Part model, mm, in its own coordinate system. Face numbers are marked on the shaded views. A direction names the side the tool comes from. Round coordinates to 2 decimals unless told otherwise and drop trailing zeros. Loops run counter-clockwise (first coordinate to the right, second up) from the corner with the lowest first, then second, coordinate; pieces in that order, holes last.
(1) Cut at B-B on z = -49. List the corners of the cut face in (x, y).
(2) Tool access for the marked faces 1 and 2: list every direction of +Z, -Z, +X, -X, +Y, -Y with a clear straight run to the whole face (end or side of a thin tool).
(3) Probe probe 1 along Z at (x, y) = (11.5, -2.75); probe 2 along Z at (x, y) = (1.5, -7.75); probe 3 along Y at (x, z) = (7.5, -108). List the from-to ranges inside material, lowest first.
(4) Flat gauge pins, fed straight in: pin 1 (4 mm diameter, centred on y = -9, z = -31.5, fed in from +X); pin 2 (2.5 mm diameter, centred on x = 6.5, y = 2.5, fed in from -Z); pin 3 (1 mm diameter, centred on y = -2.5, z = -69.5, fed in from -X); pin 4 (4 mm diameter, centred on x = 9.5, z = -116, fed in from +Y). Where does each tip first touch, or does it go through?
(5) Cut at C-C on y = 2. List the corners of the cut face in (x, z).
(6) Cut at A-A on x = 8. List the corners of the cut face in (y, z).
(7) Cut at D-D on y = -8. List the corners of the cut face in (x, z).
from build123d import *

# Parameters (mm, degrees)
BOSS_EXTRUDE1_DEPTH     = 12
SKETCH2_W               = 8
SKETCH2_H               = 75
CUT_EXTRUDE1_DEPTH      = 9
CUT_EXTRUDE1_DEPTH_BACK = 18.172456897


with BuildPart() as part:
    # Sketch1 → Boss-Extrude1 (new body)
    with BuildSketch(Plane(origin=(0, 0, 0), x_dir=(0, 0, -1), z_dir=(1, 0, 0))):
        with BuildLine():
            Line((0, 0), (0, 8))
            ThreePointArc((0, 8), (40, -12), (80, 8))
            Line((80, 8), (88, 8))
            ThreePointArc((88, 8), (106.5, 4), (125, 8))
            Line((125, 8), (145, 8))
            Line((145, 8), (145, 6))
            ThreePointArc((145, 6), (135.440306509, 1.532311637), (125, 0))
            Line((125, 0), (80, 0))
            ThreePointArc((80, 0), (40, -17.172456897), (0, 0))
        make_face()
    extrude(amount=BOSS_EXTRUDE1_DEPTH)

    # Sketch2 → Cut-Extrude1 (cut, two sides)
    with BuildSketch(Plane(origin=(0, 0, 0), x_dir=(1, 0, 0), z_dir=(0, 1, 0))) as cut_extrude1_sk:
        with Locations((6, 39.5)):
            Rectangle(SKETCH2_W, SKETCH2_H)
    extrude(amount=CUT_EXTRUDE1_DEPTH, mode=Mode.SUBTRACT)
    extrude(cut_extrude1_sk.sketch, amount=-CUT_EXTRUDE1_DEPTH_BACK, mode=Mode.SUBTRACT)


solid = part.part
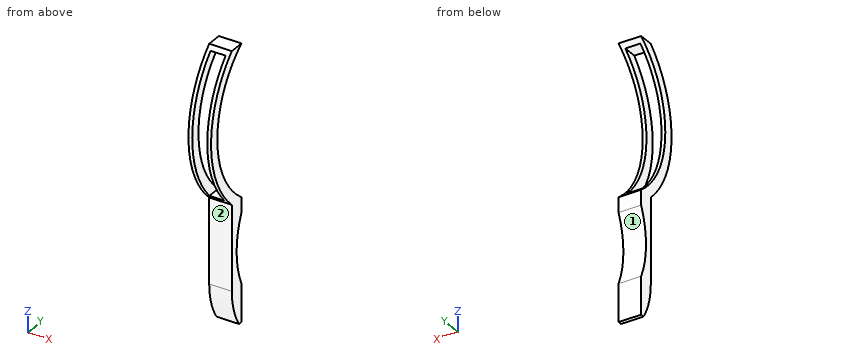
Final values:
1. outline: (0, -16.43) - (2, -16.43) - (2, -11.18) - (0, -11.18) - close; (10, -16.43) - (12, -16.43) - (12, -11.18) - (10, -11.18) - close
2. face 1: +X, -X, +Y
2. face 2: -Z, +X, -X, -Y
3. probe 1: z = -77.19 to -68.97, -11.03 to -2.81
3. probe 2: z = -70.84 to -60.17, -19.83 to -9.16
3. probe 3: y = 0 to 4.03
4. pin 1: passes through
4. pin 2: stops at z = -141.08
4. pin 3: stops at x = 0
4. pin 4: stops at y = 5.5
5. outline: (0, -136.89) - (12, -136.89) - (12, -74.7) - (10, -74.7) - (10, -77) - (2, -77) - (2, -74.7) - (0, -74.7) - close; (0, -5.3) - (2, -5.3) - (2, -2) - (10, -2) - (10, -5.3) - (12, -5.3) - (12, 0) - (0, 0) - close
6. outline: (-2.93, -77) arc R55.17 ccw to (0, -80) - (0, -125) arc R36.33 ccw to (6, -145) - (8, -145) - (8, -125) arc R44.78 cw to (8, -88) - (8, -80) arc R50 cw to (4.37, -77) - close; (-2, -2) - (5.5, -2) arc R50 cw to (8, 0) - (0, 0) arc R55.17 ccw to start
7. outline: (0, -70.46) - (2, -70.46) - (2, -59.6) - (0, -59.6) - close; (0, -20.4) - (2, -20.4) - (2, -9.54) - (0, -9.54) - close; (10, -70.46) - (12, -70.46) - (12, -59.6) - (10, -59.6) - close; (10, -20.4) - (12, -20.4) - (12, -9.54) - (10, -9.54) - close
